Verification items for the finished model (mm, model axes). A direction names the side the tool comes from. Round coordinates to 2 decimals unless told otherwise and drop trailing zeros. Write each loop counter-clockwise with the first axis right and the second up, starting at its lowest first coordinate (ties: lowest second). Pieces come first, ordered by that corner, then holes. Notation, with made-up numbers: (-12.5, 2) - (-7.5, 2) arc R17 ccw to (-7.5, 20) - close; hole circle Ø4 at (27.5, -37). An arc over 180 degrees is marked (long way). Answer as a JSON object with one key per item and string values. Group by question number.
1) Section check D-D (x = 8.25). Enter the section's corners in (y, z).
2) Go/stop test with flat-tipped pins: pin 1 Ø10 at (x, z) = (-10.5, 6) entering from -Y; pin 2 Ø6 at (y, z) = (23, -11.5) entering from +X; pin 3 Ø2 at (x, y) = (-11, 48.5) entering from -Z; pin 4 Ø12 at (y, z) = (14.5, 11) entering from -X. Record where each tip stops, or that it passes through.
3) Section check C-C (z = 28). Enter the section's corners in (x, y).
4) Section check A-A (x = 3.25). Enter the section's corners in (y, z).
5) Section check B-B (y = 21). Enter the section's corners in (x, z).
6) Thickness scan on line 1 (Z direction, x = -0.5, y = 36.5); line 2 (Y direction, x = 5.75, z = 29.5); line 3 (Z direction, x = 10.25, y = 3). Record the ranges inside material, lowest first.
7) Mould release check, pull along Y, two halves, no side actions. Record for faces 3 (the flat face through (0, 57.404, 0)), 4 (the cylindrical face through (2.93, 45.42, 27.62)), 5 (the flat face through (0, 51, -26.924)): +Y half, -Y half, draft (parallel to the pull), parting line (faces both ways), or undercut.
8) Set-up check for faces 1 (the cylindrical face through (-6.344, 51.333, -19.925)), 2 (the flat face through (0, 51, 42.926)): record each of +Z, -Z, +X, -X, +Y, -Y from which the full face is reachable in a straight line by a thin tool's end or side.
```python
from build123d import *

# Parameters (mm, degrees)
SKETCH2_R                = 14.224
BOSS_EXTRUDE1_DEPTH      = 57.404
BOSS_EXTRUDE2_DEPTH      = 28.702
BOSS_EXTRUDE2_DEPTH_BACK = 41.148
SKETCH3_R                = 6.35


with BuildPart() as part:
    # Sketch2 → Boss-Extrude1 (new body)
    with BuildSketch(Plane(origin=(0, 0, 0), x_dir=(1, 0, 0), z_dir=(0, 1, 0))):
        with Locations(Location((0, 0, 0), (0, 0, 270))):
            Circle(SKETCH2_R)
    extrude(amount=BOSS_EXTRUDE1_DEPTH)

    # Sketch3 → Boss-Extrude2 (add, two sides: drawn at the far end of the back side and taken through both)
    with BuildSketch(Plane.XY.offset(14.224).offset(-BOSS_EXTRUDE2_DEPTH_BACK)):
        with Locations((0, 51.054)):
            Circle(SKETCH3_R)
    extrude(amount=BOSS_EXTRUDE2_DEPTH + BOSS_EXTRUDE2_DEPTH_BACK)


solid = part.part
```
Returned:
{
 "1": {"outline": "(0, -11.59) - (57.4, -11.59) - (57.4, 11.59) - (0, 11.59) - close"},
 "2": {"pin 1": "y = 0", "pin 2": "x = 11.4", "pin 3": "z = -10.12", "pin 4": "x = -13.32"},
 "3": {"outline": "circle Ø12.7 at (0, 51.05)"},
 "4": {"outline": "(0, -13.85) - (45.6, -13.85) - (45.6, -26.92) - (56.51, -26.92) - (56.51, -13.85) - (57.4, -13.85) - (57.4, 13.85) - (56.51, 13.85) - (56.51, 42.93) - (45.6, 42.93) - (45.6, 13.85) - (0, 13.85) - close"},
 "5": {"outline": "circle Ø28.45 at (0, 0)"},
 "6": {"line 1": "-14.22 to 14.22", "line 2": "48.36 to 53.75", "line 3": "-9.86 to 9.86"},
 "7": {"face 3": "+Y half", "face 4": "parting line", "face 5": "draft"},
 "8": {"face 1": "-Z", "face 2": "+Z, +X, -X, +Y, -Y"}
}
